Geometry check sheet. Reference: the model listing, model coordinates, mm. Face numbers are marked on the shaded views. A direction names the side the tool comes from. Give positions to 0.01 mm unless a question says otherwise; leave off trailing zeros. Loops run counter-clockwise (first coordinate to the right, second up) from the corner with the lowest first, then second, coordinate; pieces in that order, holes last. Notation, with made-up numbers: (-30.75, -33) - (9.25, -33) arc R19 ccw to (9.25, -16) - close; hole circle Ø1 at (56.25, 79). An arc over 180 degrees is marked (long way). One line per question, with ' | ' between items. Start each with the question number.
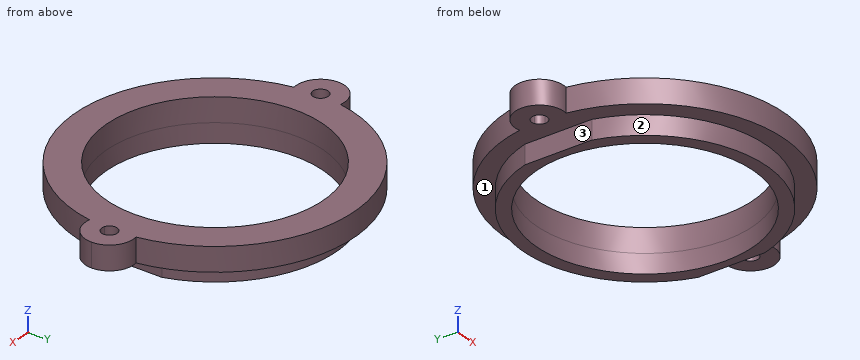
from build123d import *

# Parameters (mm, degrees)
F0_R     = 22.5
F1_DEPTH = 5
F2_DEPTH = 4


# Not quite as in the source:
# - a feature names something its author has since deleted; it is built from what else it names


with BuildPart() as f1:
    # F0 (on Top) → F1 (new body)
    with BuildSketch(Plane.XY):
        with BuildLine():
            ThreePointArc((28.5805084746, -4.9147263743), (24.5, 0), (28.5805084746, 4.9147263743))
            ThreePointArc((28.5805084746, 4.9147263743), (0, 29), (-28.5805084746, 4.9147263743))
            ThreePointArc((-28.5805084746, 4.9147263743), (-25.6530884058, 3.1939428903), (-24.5, 0))
            ThreePointArc((-24.5, 0), (-25.6530884058, -3.1939428903), (-28.5805084746, -4.9147263743))
            ThreePointArc((-28.5805084746, -4.9147263743), (0, -29), (28.5805084746, -4.9147263743))
        make_face()
        with BuildLine():
            ThreePointArc((-24.24, 7.07), (0, 25.25), (24.24, 7.07))
            Line((24.24, 7.07), (24.24, -7.07))
            ThreePointArc((24.24, -7.07), (0, -25.25), (-24.24, -7.07))
            Line((-24.24, -7.07), (-24.24, 7.07))
        make_face(mode=Mode.SUBTRACT)
        with BuildLine():
            Line((24.24, -7.07), (24.24, 7.07))
            ThreePointArc((24.24, 7.07), (0, 25.25), (-24.24, 7.07))
            Line((-24.24, 7.07), (-24.24, -7.07))
            ThreePointArc((-24.24, -7.07), (0, -25.25), (24.24, -7.07))
        make_face()
        Circle(F0_R, mode=Mode.SUBTRACT)
        with BuildLine():
            ThreePointArc((-28.9608474576, 1.506424421), (-28.8211040937, 3.2162025464), (-28.5805084746, 4.9147263743))
            ThreePointArc((-28.5805084746, 4.9147263743), (-34.5, 0), (-28.5805084746, -4.9147263743))
            ThreePointArc((-28.5805084746, -4.9147263743), (-28.8211040937, -3.2162025464), (-28.9608474576, -1.506424421))
            ThreePointArc((-28.9608474576, -1.506424421), (-31.1, 0), (-28.9608474576, 1.506424421))
        make_face()
        with BuildLine():
            ThreePointArc((28.5805084746, 4.9147263743), (28.8211040937, 3.2162025464), (28.9608474576, 1.506424421))
            ThreePointArc((28.9608474576, 1.506424421), (30.4212371932, 1.3081750777), (31.1, 0))
            ThreePointArc((31.1, 0), (30.4212371932, -1.3081750777), (28.9608474576, -1.506424421))
            ThreePointArc((28.9608474576, -1.506424421), (28.8211040937, -3.2162025464), (28.5805084746, -4.9147263743))
            ThreePointArc((28.5805084746, -4.9147263743), (32.6939428903, -3.8469115942), (34.5, 0))
            ThreePointArc((34.5, 0), (32.6939428903, 3.8469115942), (28.5805084746, 4.9147263743))
        make_face()
        with BuildLine():
            ThreePointArc((-24.5, 0), (-25.6530884058, 3.1939428903), (-28.5805084746, 4.9147263743))
            ThreePointArc((-28.5805084746, 4.9147263743), (-28.8211040937, 3.2162025464), (-28.9608474576, 1.506424421))
            ThreePointArc((-28.9608474576, 1.506424421), (-28.1918249223, 0.9212371932), (-27.9, 0))
            ThreePointArc((-27.9, 0), (-28.1918249223, -0.9212371932), (-28.9608474576, -1.506424421))
            ThreePointArc((-28.9608474576, -1.506424421), (-28.8211040937, -3.2162025464), (-28.5805084746, -4.9147263743))
            ThreePointArc((-28.5805084746, -4.9147263743), (-25.6530884058, -3.1939428903), (-24.5, 0))
        make_face()
        with BuildLine():
            ThreePointArc((28.9608474576, -1.506424421), (27.9, 0), (28.9608474576, 1.506424421))
            ThreePointArc((28.9608474576, 1.506424421), (28.8211040937, 3.2162025464), (28.5805084746, 4.9147263743))
            ThreePointArc((28.5805084746, 4.9147263743), (24.5, 0), (28.5805084746, -4.9147263743))
            ThreePointArc((28.5805084746, -4.9147263743), (28.8211040937, -3.2162025464), (28.9608474576, -1.506424421))
        make_face()
    extrude(amount=F1_DEPTH)

    # F0 (on Top) → F2 (join)
    with BuildSketch(Plane.XY):
        with BuildLine():
            Line((24.24, -7.07), (24.24, 7.07))
            ThreePointArc((24.24, 7.07), (0, 25.25), (-24.24, 7.07))
            Line((-24.24, 7.07), (-24.24, -7.07))
            ThreePointArc((-24.24, -7.07), (0, -25.25), (24.24, -7.07))
        make_face()
        Circle(F0_R, mode=Mode.SUBTRACT)
    extrude(amount=-F2_DEPTH)


solid = f1.part
(1) Section check D-D, the plane z = 3.75. Record the boundary of the cut face in (x, y).
(2) Tool access check on the marked faces 1, 2 and 3. Record the directions out of +Z, -Z, +X, -X, +Y, -Y that give a thin tool (end or side, any length) a straight path to the whole face; none if there is none.
(3) Section check C-C, the plane z = -1.5. Record the boundary of the cut face in (x, y), and give its area (3 significant figures).
(4) Depth check by flat-ended pin: pin 1 Ø2 at (x, z) = (-18, -2.5) entering from +Y; pin 2 Ø1.5 at (y, z) = (17, -1) entering from -X; pin 3 Ø3 at (y, z) = (1.5, -3) entering from -X. Enter the tip coordinate at first touch or a pass-through.
(5) Section check B-B, the plane y = 17. Record the boundary of the cut face in (x, z).
(6) Section check A-A, the plane x = 0. Record the boundary of the cut face in (y, z).
(7) Material ranges on line 1 (Y direction, x = -0.5, z = -0.5); line 2 (Z direction, x = -12, y = 26); line 3 (X direction, y = 7, z = 3.25), recorded low to high.
Numbers:
1) outline: (-28.58, -4.91) arc R29 ccw to (28.58, -4.91) arc R5 ccw (long way) to (28.58, 4.91) arc R29 ccw to (-28.58, 4.91) arc R5 ccw (long way) to start; hole circle Ø3.2 at (-29.5, 0); hole circle Ø45 at (0, 0); hole circle Ø3.2 at (29.5, 0)
2) face 1: -Z | face 2: -Z, -Y | face 3: -Z, -X, +Y, -Y
3) outline: (-24.24, -7.07) arc R25.25 ccw to (24.24, -7.07) - (24.24, 7.07) arc R25.25 ccw to (-24.24, 7.07) - close; hole circle Ø45 at (0, 0) | area: 393 mm^2
4) pin 1: y = 18.67 | pin 2: x = -19.33 | pin 3: x = -24.24
5) outline: (-23.49, 0) - (-18.67, 0) - (-18.67, -4) - (-14.74, -4) - (-14.74, 5) - (-23.49, 5) - close; (14.74, -4) - (18.67, -4) - (18.67, 0) - (23.49, 0) - (23.49, 5) - (14.74, 5) - close
6) outline: (-29, 0) - (-25.25, 0) - (-25.25, -4) - (-22.5, -4) - (-22.5, 5) - (-29, 5) - close; (22.5, -4) - (25.25, -4) - (25.25, 0) - (29, 0) - (29, 5) - (22.5, 5) - close
7) line 1: -25.25 to -22.49, 22.49 to 25.25 | line 2: 0 to 5 | line 3: -28.14 to -21.38, 21.38 to 28.14
